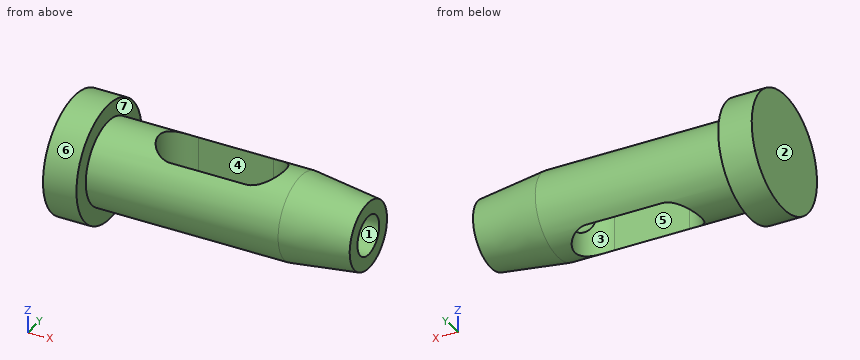
```python
from build123d import *

# Parameters (mm, degrees)
F3_DEPTH      = 21.001
F3_DEPTH_BACK = 21.001
F4_R          = 7
F5_DEPTH      = 34.3431458505


with BuildPart() as f1:
    # F0 (on Front) → F1 (revolve)
    with BuildSketch(Plane.XZ):
        Polygon((-105, 21), (-105, 0), (0, 0), (0, 12), (-24, 15), (-93, 15), (-93, 21), align=None)
    revolve(axis=Axis((-52.5, 0, 0), (1, 0, 0)))

    # F2 (on Top) → F3 (cut, two sides)
    with BuildSketch(Plane.XY) as f3_sk:
        with BuildLine():
            ThreePointArc((-39, -9), (-30, 0), (-39, 9))
            Line((-39, 9), (-66, 9))
            ThreePointArc((-66, 9), (-75, 0), (-66, -9))
            Line((-66, -9), (-39, -9))
        make_face()
    extrude(amount=-F3_DEPTH, mode=Mode.SUBTRACT)
    extrude(f3_sk.sketch, amount=F3_DEPTH_BACK, mode=Mode.SUBTRACT)

    # F4 (on face) → F5 (cut, up to face)
    with BuildSketch(Plane.YZ):
        Circle(F4_R)
    extrude(amount=-F5_DEPTH, mode=Mode.SUBTRACT)


solid = f1.part
```
Could you check a few things on this model? Use its own coordinates, in mm. Face numbers are marked on the shaded views. A direction names the side the tool comes from. Give positions to 0.01 mm unless a question says otherwise; leave off trailing zeros. Loops run counter-clockwise (first coordinate to the right, second up) from the corner with the lowest first, then second, coordinate; pieces in that order, holes last. Notation, with made-up numbers: (72, -20) - (84, -20) arc R24 ccw to (84, -4) - close; hole circle Ø10 at (50, 27). An arc over 180 degrees is marked (long way). Answer in a Markdown table with one row per item. Add a question column.
Q1. For pin 1 (7 mm diameter, centred on x = -50.5, z = -4.5, fed in from +Y); pin 2 (4 mm diameter, centred on x = -29, y = -6.5, fed in from +Z); pin 3 (2 mm diameter, centred on y = -17, z = 6.5, fed in from +X), each with a flat end and sliding along its axis, tell me the tip position at first contact or that it passes through.
Q2. Please list where these lines run through material, in increasing order: L1, parallel to Y at x = -24.5, z = 0; L2, parallel to X at y = -14, z = 15. Write a range as from..to.
Q3. If we section it at D-D (x = -88): List the corners of the cut face in (y, z) for me.
Q4. If we section it at B-B (z = 0): List the corners of the cut face in (x, y) for me.
Q5. Which directions (+Z, -Z, +X, -X, +Y, -Y) give clear straight access to the entire face, cutting with the end or side of a thin tool? Please do the marked faces 1, 2 and 3.
Q6. If we section it at C-C (x = -47): List the corners of the cut face in (y, z) for me, plus the area to 3 significant figures.
Q7. If we section it at A-A (y = 0): List the corners of the cut face in (x, z) for me.
Q8. We'd pull the mould along Y, two halves only. Please class the marked faces 4, 5, 6 and 7: +Y half, -Y half, draft (parallel to the pull), parting line (faces both ways), or undercut.
The answers:
| question | item | result |
|---|---|---|
| 1 | pin 1 | stops at y = 14.97 |
| 1 | pin 2 | stops at z = 14.31 |
| 1 | pin 3 | stops at x = -93 |
| 2 | L1 | y = -15..-7, 7..15 |
| 2 | L2 | x = -105..-93 |
| 3 | outline | circle Ø30 at (0, 0) |
| 4 | outline | (-105, -21) - (-93, -21) - (-93, -15) - (-24, -15) - (0, -12) - (0, -7) - (-33.34, -7) arc R9 cw to (-39, -9) - (-66, -9) arc R9 cw to (-66, 9) - (-39, 9) arc R9 cw to (-33.34, 7) - (0, 7) - (0, 12) - (-24, 15) - (-93, 15) - (-93, 21) - (-105, 21) - close |
| 5 | face 1 | +X |
| 5 | face 2 | +Z, -Z, -X, +Y, -Y |
| 5 | face 3 | +Z, -Z |
| 6 | outline | (-9, -12) - (-9, 12) arc R15 ccw to start; (9, -12) arc R15 ccw to (9, 12) - close |
| 6 | area | 201 mm^2 |
| 7 | outline | (-105, -21) - (-93, -21) - (-93, -15) - (-75, -15) - (-75, 15) - (-93, 15) - (-93, 21) - (-105, 21) - close; (-30, -15) - (-24, -15) - (0, -12) - (0, -7) - (-30, -7) - close; (-30, 7) - (0, 7) - (0, 12) - (-24, 15) - (-30, 15) - close |
| 8 | face 4 | undercut |
| 8 | face 5 | undercut |
| 8 | face 6 | parting line |
| 8 | face 7 | draft |
